Autodesk Inventor part; units mm, degrees
ref_plane "YZ Plane" through (0, 0, 0) normal (1, 0, 0) x (0, 1, 0)
ref_plane "XZ Plane" through (0, 0, 0) normal (0, 1, 0) x (-1, 0, 0)
ref_plane "XY Plane" through (0, 0, 0) normal (0, 0, 1) x (1, 0, 0)
sketch "Boceto1" plane through (0, 0, 0) normal (0, 1, 0) x (-1, 0, 0)
  circle A0 centre (0, 0) radius 17.05
  circle A1 centre (0, 0) radius 19.05
  dimension "d0" = 34.1
  dimension "d1" = 38.1
extrude "Extrusión1" add sketch "Boceto1" along normal blind 813.6
sketch "Boceto2" plane through (0, 0, 0) normal (0, 0, 1) x (1, 0, 0)
  line L0 (0, 0) -> (-263.1264, 0)
  line L1 (-263.1264, 0) -> (-263.1264, 271)
  line L2 (-263.1264, 135.5) -> (-17.2798, 135.5)
  line L3 (-19.05, 0) -> (-19.05, 813.6)
  line L4 (-17.2798, 135.5) -> (-17.2798, 51.5895)
  line L5 (-17.2798, 51.5895) -> (12.7202, 51.5895)
  line L6 (12.7202, 51.5895) -> (12.7202, 21.5895)
  line L7 (12.7202, 21.5895) -> (-17.2798, 21.5895)
  line L8 (-17.2798, 21.5895) -> (-17.2798, 51.5895)
  dimension "d4" = 271
  dimension "d5" = 30
  dimension "d6" = 30
extrude "Extrusión2" cut sketch "Boceto2" against normal blind 813.6 contours L5 L6 L7 L8
sketch "Boceto3" plane through (0, 813.6, 0) normal (0, 1, 0) x (1, 0, 0)
  circle A0 centre (0, 0) radius 27.5
  circle A1 centre (0, 0) radius 19.05
  dimension "d9" = 55
extrude "Extrusión3" add sketch "Boceto3" against normal blind 3 contours A0 | A1
sketch "Boceto4" plane through (0, 813.6, 0) normal (0, 1, 0) x (1, 0, 0)
  circle A0 centre (0, 0) radius 17.05
  circle A1 centre (0, 0) radius 27.5
  line L0 (0, 0) -> (0, 23.75)
  line L1 (0, 0) -> (23.75, 0)
  line L2 (0, 0) -> (0, -23.75)
  line L3 (0, 0) -> (-23.75, 0)
  circle A2 centre (0, 23.75) radius 2.75
  circle A3 centre (23.75, 0) radius 2.75
  circle A4 centre (0, -23.75) radius 2.75
  circle A5 centre (-23.75, 0) radius 2.75
  dimension "d22" = 23.75
  dimension "d23" = 23.75
  dimension "d24" = 23.75
  dimension "d25" = 23.75
  dimension "d26" = 5.5
  dimension "d27" = 5.5
  dimension "d28" = 5.5
  dimension "d29" = 5.5
extrude "Extrusión4" cut sketch "Boceto4" against normal blind 5.5 contours A4 | A5 | A2 | A3
sketch "Boceto5" plane through (0, 813.6, 0) normal (0, 1, 0) x (1, 0, 0)
  circle A0 centre (0, 0) radius 17.05
  dimension "d19" = 34.1
extrude "Extrusión5" cut sketch "Boceto5" against normal blind 3
equation "\"d17\" = d27"
properties part number "tubo cubierta tornillo"
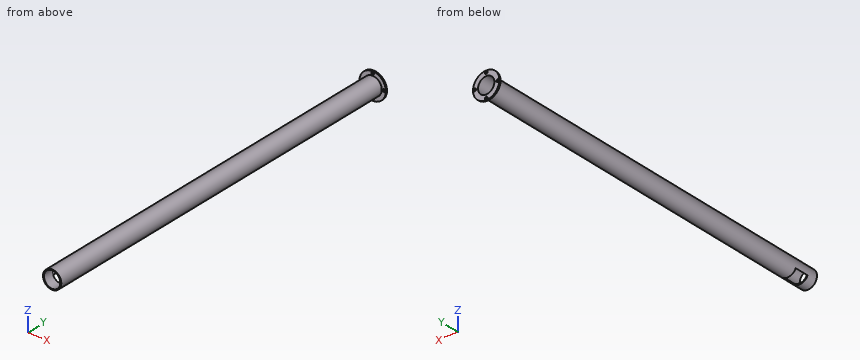
Here's how the part is built. I have some questions about the finished solid (model axes, mm). Give positions to 0.01 mm unless a question says otherwise; leave off trailing zeros. Loops run counter-clockwise (first coordinate to the right, second up) from the corner with the lowest first, then second, coordinate; pieces in that order, holes last. Notation, with made-up numbers: (5, 77) -> (64, 77) arc R13 ccw to (64, 92) -> close; hole circle Ø2 at (42.5, 5.25). An arc over 180 degrees is marked (long way). One line per item, written item: value.
Q1. I'm going to push flat-ended pins straight in: pin 1 Ø4 at (x, z) = (1, -16) entering from -Y; pin 2 Ø5 at (x, y) = (16.5, 199) entering from -Z; pin 3 Ø0.8 at (y, z) = (34, -13) entering from -X; pin 4 Ø5 at (y, z) = (730.5, 13) entering from +X. Where does each tip first touch, or does it pass through?
Answers follow:
pin 1: y = 0
pin 2: z = -12.92
pin 3: x = 12.72
pin 4: x = 15.9
Q2. Suppose I cut it at A-A on y = 591. Please give me the cut outline in (x, z).
Answers follow:
outline: circle Ø38.1 at (0, 0); hole circle Ø34.1 at (0, 0)
Q3. If I drill on line 1 along Z through (x, y) = (0, 811); line 2 along X through (y, z) = (552, 0), over which ranges is the centre line in solid material (lowest first)?
Answers follow:
line 1: -27.5 to -26.5, -21 to -17.05, 17.05 to 21, 26.5 to 27.5
line 2: -19.05 to -17.05, 17.05 to 19.05
